Geometry: final body of the model. Coordinates: model frame, mm. Face numbers are marked on the shaded views. A direction names the side the tool comes from. Round coordinates to 2 decimals unless told otherwise and drop trailing zeros. Order: outer loops, then holes, each group sorted by start corner. A loop starts at its lowest first (then second) coordinate and runs counter-clockwise, first axis right, second up. Notation, with made-up numbers: M 9,49.5 L 41,49.5 A19 cw 41,59.5 Z; hole C 7,44 d9. An arc over 180 degrees is marked long. Return JSON: item names as keys, results as strings. Group by question number.
Q1. Mould query, pull axis Z, two halves, no side actions, for the marked faces 4, 5, 6 and 7. Classes: released by +Z, released by -Z, zero draft, split by the parting line, or undercut.
Q2. Cut plane C-C on y = 0. Output: boundary loops of the cut face in (x, z), and give its area (3 significant figures).
Q3. Ray query, probe 1 along X at (y, z) = (-2.5, 7); probe 2 along Z at (x, y) = (8.5, -1.7); probe 3 along Z at (x, y) = (8.5, -3.15). Return the intervals inside material, ascending.
Q4. Contact query for flat-ended pins moving along their axis: pin 1 (5.5 mm diameter, centred on x = 7, z = 6.5, fed in from +Y); pin 2 (6 mm diameter, centred on x = 0, z = -4, fed in from +Y); pin 3 (8 mm diameter, centred on x = 0, y = 3.5, fed in from +Z). Output: stop coordinate, or through.
Q5. Cut plane B-B on x = 8.5. Output: boundary loops of the cut face in (y, z), and give its area (3 significant figures).
Q6. Cut plane D-D on x = 1. Output: boundary loops of the cut face in (y, z).
Q7. Cut plane A-A on z = 0. Output: boundary loops of the cut face in (x, y).
Q8. Access query for the marked faces 1, 2 and 3. Directions: +Z, -Z, +X, -X, +Y, -Y. A direction counts if a zero-diameter tool reaches every point of the face in a straight line with its end or side. Return the directions, or none.
Autodesk Inventor part; units mm, degrees
ref_plane "part1_to_part2_XY" through (5, 0, 0) normal (1, 0, 0) x (0, 0, -1)
ref_plane "part1_to_part2_YZ" through (5, 0, 0) normal (0, 0, -1) x (0, 1, 0)
ref_plane "part1_to_part2_ZX" through (5, 0, 0) normal (0, 1, 0) x (1, 0, 0)
sketch "Sketch_1" plane through (0, 0, 0) normal (0, 0, 1) x (1, 0, 0)
  line L0 (5, 0) -> (-5, 0)
  line L1 (-5, 0) -> (-5, 12.5)
  line L2 (-5, 12.5) -> (-2.6142, 12.5)
  line L3 (-2.6142, 12.5) -> (-1.3716, 9.5)
  line L4 (-1.3716, 9.5) -> (1.3716, 9.5)
  line L5 (1.3716, 9.5) -> (2.6142, 12.5)
  line L6 (2.6142, 12.5) -> (5, 12.5)
  line L7 (5, 12.5) -> (5, 0)
  line L8 (5, 0) -> (-5, 0)
revolve "Revolution1" add sketch "Sketch_1" angle 360 about axis through (5, 0, 0) along (1, 0, 0)
sketch "Sketch_2" plane through (0, 0, 0) normal (0, 0, 1) x (1, 0, 0)
  line L0 (5, 0) -> (11, 0)
  line L1 (11, 0) -> (11, -9.5)
  line L2 (11, -9.5) -> (10.5, -10)
  line L3 (10.5, -10) -> (5, -10)
  line L4 (5, -10) -> (5, 0)
  line L5 (5, 0) -> (11, 0)
revolve "Revolution2" add sketch "Sketch_2" angle 180 mid plane about axis through (5, 0, 0) along (1, 0, 0)
sketch "Sketch_3" plane through (0, 0, 0) normal (0, 0, 1) x (1, 0, 0)
  line L0 (5, -0.5) -> (11, -0.5)
  line L1 (11, -0.5) -> (11, 0)
  line L2 (11, 0) -> (5, 0)
  line L3 (5, 0) -> (5, -0.5)
extrude "Extrusion1" cut sketch "Sketch_3" along normal mid plane 40
sketch "Sketch_9" plane through (8.5, 0, 0) normal (1, 0, 0) x (0, 0, -1)
  line L0 (7, -10) -> (7, -0.5)
  line L1 (7, -0.5) -> (8.5, -0.5)
  line L2 (8.5, -0.5) -> (8.2295, -0.7705)
  line L3 (8.2295, -0.7705) -> (8.2295, -9.7295)
  line L4 (8.2295, -9.7295) -> (8.5, -10)
  line L5 (8.5, -10) -> (7, -10)
  line L6 (7, -10) -> (7, -0.5)
revolve "Revolution4" cut sketch "Sketch_9" angle 360 about axis through (8.5, -10, -7) along (0, -1, 0)
sketch "Sketch_6" plane through (8.5, 0, 0) normal (1, 0, 0) x (0, 0, -1)
  line L0 (-7, -10) -> (-7, -0.5)
  line L1 (-7, -0.5) -> (-5.5, -0.5)
  line L2 (-5.5, -0.5) -> (-5.7705, -0.7705)
  line L3 (-5.7705, -0.7705) -> (-5.7705, -9.7295)
  line L4 (-5.7705, -9.7295) -> (-5.5, -10)
  line L5 (-5.5, -10) -> (-7, -10)
  line L6 (-7, -10) -> (-7, -0.5)
revolve "Revolution5" cut sketch "Sketch_6" angle 360 about axis through (8.5, -10, 7) along (0, -1, 0)
ref_plane "part1_to_part2_XY" through (5, 0, 0) normal (1, 0, 0) x (0, 0, -1)
ref_plane "part1_to_part2_YZ" through (5, 0, 0) normal (0, 0, -1) x (0, 1, 0)
ref_plane "part1_to_part2_ZX" through (5, 0, 0) normal (0, 1, 0) x (1, 0, 0)
sketch "スケッチ7" plane through (-5, 0, 0) normal (-1, 0, 0) x (0, 0, 1)
  circle A0 centre (0, 0) radius 5.1
  dimension "d12" = 10.2
extrude "押し出し2" cut sketch "スケッチ7" against normal through all
ref_plane "作業平面4" through (7.75, -10, 0) normal (0, 1, 0) x (-1, 0, 0)
sketch "スケッチ8" plane through (7.75, -10, 0) normal (0, 1, 0) x (-1, 0, 0)
  circle A0 centre (-0.75, 7) radius 1.2295
  circle A1 centre (-0.75, 7) radius 1.7
  circle A2 centre (-0.75, -7) radius 1.5
  circle A3 centre (-0.75, -7) radius 1.7
  circle A4 centre (-0.75, 7) radius 3.5
  circle A5 centre (-0.75, -7) radius 3.5
  point P0 (7.75, 0)
  dimension "d15" = 3.4
  dimension "d16" = 3.4
  dimension "d17" = 7
  dimension "d18" = 7
extrude "押し出し3" cut sketch "スケッチ8" along normal through all contours A0 | A1 | A2 | A3
extrude "押し出し4" cut sketch "スケッチ8" along normal blind 5 contours A0 | A1 | A2 | A3 | A4 | A5
properties part number "MBRDAC23-2-8_p1"
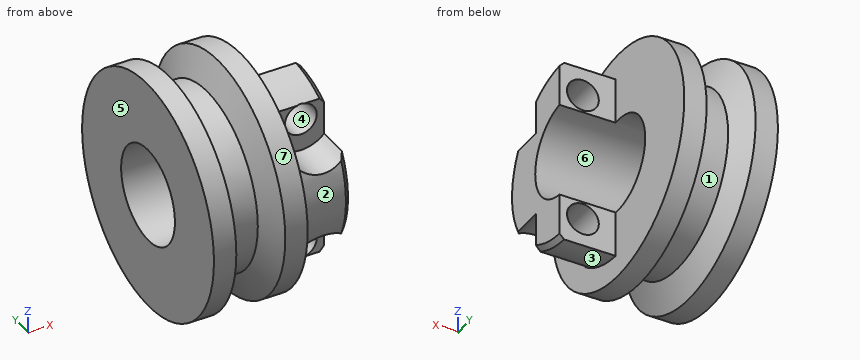
Result sheet:
{
 "1": {"face 4": "undercut", "face 5": "zero draft", "face 6": "undercut", "face 7": "split by the parting line"},
 "2": {"outline": "M -5,-12.5 L -2.61,-12.5 L -1.37,-9.5 L 1.37,-9.5 L 2.61,-12.5 L 5,-12.5 L 5,-5.1 L -5,-5.1 Z; M -5,5.1 L 5,5.1 L 5,12.5 L 2.61,12.5 L 1.37,9.5 L -1.37,9.5 L -2.61,12.5 L -5,12.5 Z", "area": "124 mm²"},
 "3": {"probe 1": "x = -5 to 6.8, 10.2 to 11", "probe 2": "z = -9.85 to -8.7, -5.3 to -4.81, 4.81 to 5.3, 8.7 to 9.85", "probe 3": "z = -9.49 to -8.7, -5.3 to -4.01, 4.01 to 5.3, 8.7 to 9.49"},
 "4": {"pin 1": "stops at y = 11.62", "pin 2": "stops at y = 12.24", "pin 3": "stops at z = 12.49"},
 "5": {"outline": "M -9.37,-3.5 L -5,-3.5 L -5,-5.3 L -0.5,-5.3 L -0.5,-5.08 A5.1 cw -0.5,5.08 L -0.5,5.3 L -5,5.3 L -5,3.5 L -9.37,3.5 A10 ccw Z; M -4.93,-8.7 A10 ccw -0.5,-9.99 L -0.5,-8.7 Z; M -4.93,8.7 L -0.5,8.7 L -0.5,9.99 A10 ccw Z", "area": "52.8 mm²"},
 "6": {"outline": "C 0,0 d19; hole C 0,0 d10.2"},
 "7": {"outline": "M -5,-12.5 L -2.61,-12.5 L -1.37,-9.5 L 1.37,-9.5 L 2.61,-12.5 L 5,-12.5 L 5,-10 L 10.5,-10 L 11,-9.5 L 11,-5.1 L -5,-5.1 Z; M -5,5.1 L 5,5.1 L 5,12.5 L 2.61,12.5 L 1.37,9.5 L -1.37,9.5 L -2.61,12.5 L -5,12.5 Z"},
 "8": {"face 1": "none", "face 2": "+X, -Y", "face 3": "-Z, +X, -Y"}
}
